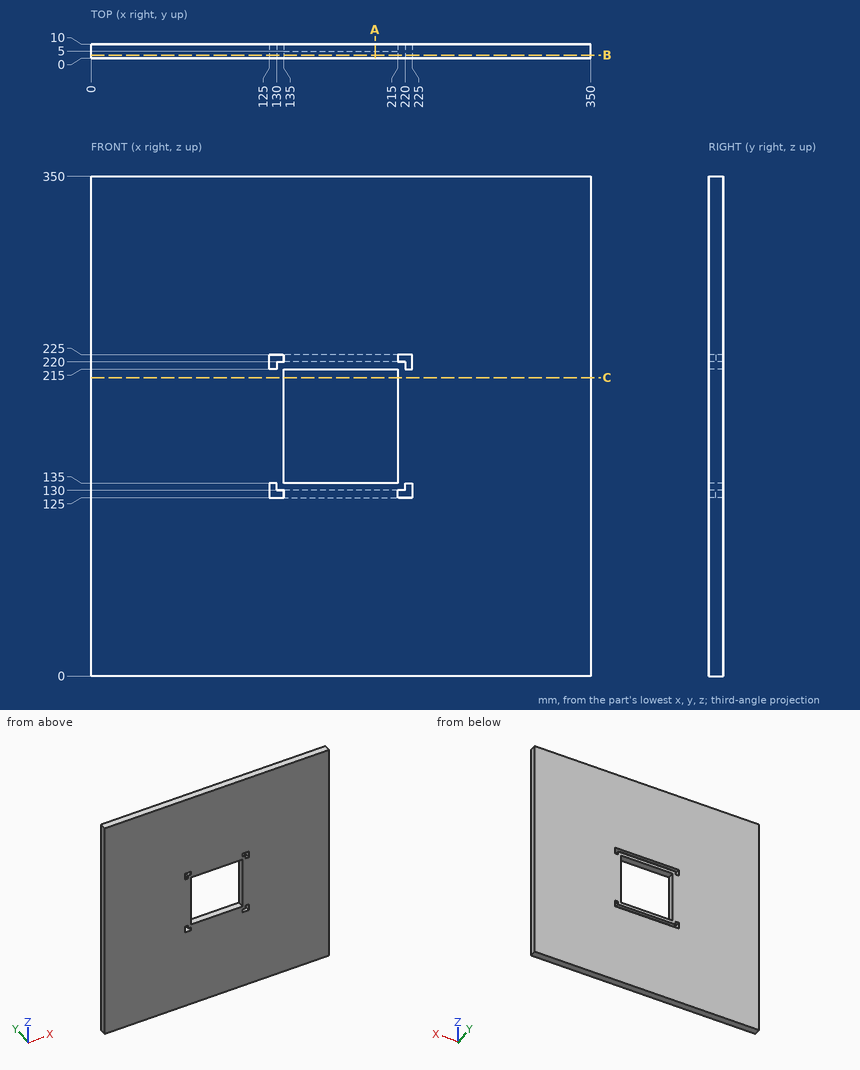
Geometry: see drawing. Coordinates: mm, zero at the bounding-box minimum. Coordinates: 2 decimals unless noted, no trailing zeros. Write each loop counter-clockwise with the first axis right and the second up, starting at its lowest first coordinate (ties: lowest second). Pieces come first, ordered by that corner, then holes. Notation, with made-up numbers: M 74,22 L 129,22 A23 cw 129,32 Z; hole C -36,53.25 d7. An arc over 180 degrees is marked long. Use CSV: the item, a comma, the result in double quotes. Start each with the question number.
1. Cut plane A-A on x = 199. Return the cut outline in (y, z), plus the area to 3 significant figures.
2. Cut plane C-C on z = 209. Return the cut outline in (x, y).
3. Ray query, probe 1 along Z at (x, y) = (210.5, 7); probe 2 along Z at (x, y) = (221, 4.5); probe 3 along Z at (x, y) = (173, 1.25). Return the intervals inside material, ascending.
4. Cut plane B-B on y = 2.25. Count the separate pieces of the cut face and the enclosed holes in it, plus the area to 3 significant figures.
Entries:
1,outline,"M 0,0 L 10,0 L 10,125 L 5,125 L 5,130 L 10,130 L 10,135 L 0,135 Z; M 0,215 L 10,215 L 10,220 L 5,220 L 5,225 L 10,225 L 10,350 L 0,350 Z"
1,area,"2,650 mm²"
2,outline,"M 0,0 L 135,0 L 135,10 L 0,10 Z; M 215,0 L 350,0 L 350,10 L 215,10 Z"
3,probe 1,"0 to 125, 130 to 135, 215 to 220, 225 to 350"
3,probe 2,"0 to 125, 135 to 215, 225 to 350"
3,probe 3,"0 to 135, 215 to 350"
4,separate pieces,"1"
4,enclosed holes,"5"
4,area,"116,000 mm²"
